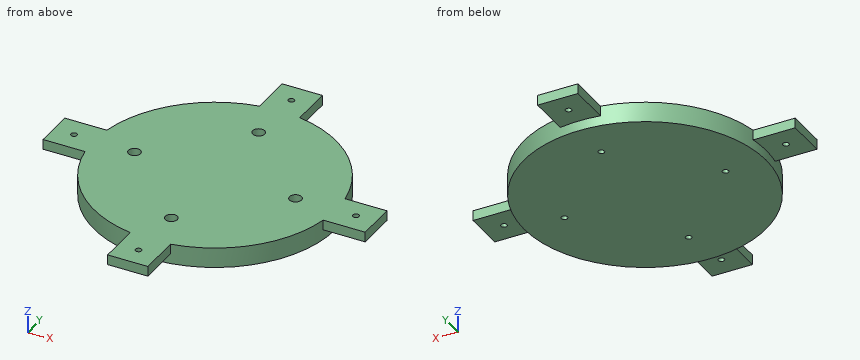
```python
from build123d import *

# Parameters (mm, degrees)
SKETCH1_R           = 60
BOSS_EXTRUDE1_DEPTH = 5
SKETCH3_W           = 20
SKETCH3_H           = 30
SKETCH3_W_2         = 30
SKETCH3_H_2         = 20
BOSS_EXTRUDE2_DEPTH = 5
SKETCH6_R           = 60
BOSS_EXTRUDE3_DEPTH = 10
SKETCH7_R           = 70
CUT_EXTRUDE2_DEPTH  = 5
SKETCH8_R           = 3
CUT_EXTRUDE7_DEPTH  = 5
SKETCH13_R          = 1.5
CUT_EXTRUDE10_DEPTH = 10


with BuildPart() as part:
    # Sketch1 → Boss-Extrude1 (new body)
    with BuildSketch(Plane.XY):
        Circle(SKETCH1_R)
    extrude(amount=BOSS_EXTRUDE1_DEPTH)

    # Sketch3 → Boss-Extrude2 (add)
    with BuildSketch(Plane(origin=(0, 0, 0), x_dir=(-1, 0, 0), z_dir=(0, 0, -1))):
        with Locations((0, -65)):
            Rectangle(SKETCH3_W, SKETCH3_H)
        with Locations((0, 65)):
            Rectangle(SKETCH3_W, SKETCH3_H)
        with Locations((65, 0)):
            Rectangle(SKETCH3_W_2, SKETCH3_H_2)
        with Locations((-65, 0)):
            Rectangle(SKETCH3_W_2, SKETCH3_H_2)
    extrude(amount=BOSS_EXTRUDE2_DEPTH)

    # Sketch6 → Boss-Extrude3 (add)
    with BuildSketch(Plane(origin=(0, 0, 0), x_dir=(-1, 0, 0), z_dir=(0, 0, -1))):
        Circle(SKETCH6_R)
    extrude(amount=BOSS_EXTRUDE3_DEPTH)

    # Sketch7 → Cut-Extrude2 (cut)
    with BuildSketch(Plane.XY.offset(5)):
        Circle(SKETCH7_R)
    extrude(amount=-CUT_EXTRUDE2_DEPTH, mode=Mode.SUBTRACT)

    # Sketch8 → Cut-Extrude7 (cut)
    with BuildSketch(Plane.XY):
        with Locations((0, -40)):
            Circle(SKETCH8_R)
        with Locations((0, 40)):
            Circle(SKETCH8_R)
        with Locations((-40, 0)):
            Circle(SKETCH8_R)
        with Locations((40, 0)):
            Circle(SKETCH8_R)
    extrude(amount=-CUT_EXTRUDE7_DEPTH, mode=Mode.SUBTRACT)

    # Sketch13 → Cut-Extrude10 (cut)
    with BuildSketch(Plane.XY):
        with Locations((-40, 0)):
            Circle(SKETCH13_R)
        with Locations((40, 0)):
            Circle(SKETCH13_R)
        with Locations((-70, 0)):
            Circle(SKETCH13_R)
        with Locations((70, 0)):
            Circle(SKETCH13_R)
        with Locations((0, -40)):
            Circle(SKETCH13_R)
        with Locations((0, -70)):
            Circle(SKETCH13_R)
        with Locations((0, 40)):
            Circle(SKETCH13_R)
        with Locations((0, 70)):
            Circle(SKETCH13_R)
    extrude(amount=-CUT_EXTRUDE10_DEPTH, mode=Mode.SUBTRACT)


solid = part.part
```
The model under review builds one solid part; all positions refer to its coordinate system, in mm. Round coordinates to 2 decimals unless told otherwise and drop trailing zeros. Order: outer loops, then holes, each group sorted by start corner. A loop starts at its lowest first (then second) coordinate and runs counter-clockwise, first axis right, second up. Notation, with made-up numbers: (-6.5, -30) -> (10.5, -30) arc R32 ccw to (10.5, 7) -> close; hole circle Ø7 at (61, 9). An arc over 180 degrees is marked (long way). Use a Markdown table: item, result.
Q1. We need section A-A on z = -7.5. Write out the cut boundary in (x, y), then the cut area to 3 significant figures.
Values:
| item | result |
|---|---|
| outline | circle Ø120 at (0, 0); hole circle Ø3 at (-40, 0); hole circle Ø3 at (0, -40); hole circle Ø3 at (0, 40); hole circle Ø3 at (40, 0) |
| area | 11,300 mm^2 |
Q2. For line 1 (X direction, y = 70, z = -3.1); line 2 (Y direction, x = 2.5, z = -2.25), list the stretches that pass through material, from the lowest coordinate up.
Values:
| item | result |
|---|---|
| line 1 | x = -10 to -1.5, 1.5 to 10 |
| line 2 | y = -80 to -41.66, -38.34 to 38.34, 41.66 to 80 |
Q3. Clearance check with flat-ended pins moving along their axes: P1, Ø4, axis at x = -32.5, z = -7, coming from the -Y side; P2, Ø16, axis at x = -70.5, y = 1, coming from the -Z side; P3, Ø5, axis at x = 26.5, z = -1, coming from the +Y side. State where each tip first meets the part, or that it passes through.
Values:
| item | result |
|---|---|
| P1 | stops at y = -51.67 |
| P2 | stops at z = -5 |
| P3 | stops at y = 54.99 |
Q4. We need section D-D on y = -24.5. Write out the cut boundary in (x, z).
Values:
| item | result |
|---|---|
| outline | (-54.77, -10) -> (54.77, -10) -> (54.77, 0) -> (-54.77, 0) -> close |
Q5. We need section B-B on y = -5.5. Write out the cut boundary in (x, z).
Values:
| item | result |
|---|---|
| outline | (-80, -5) -> (-59.75, -5) -> (-59.75, -10) -> (59.75, -10) -> (59.75, -5) -> (80, -5) -> (80, 0) -> (-80, 0) -> close |
Q6. We need section C-C on x = -8. Write out the cut boundary in (y, z).
Values:
| item | result |
|---|---|
| outline | (-80, -5) -> (-59.46, -5) -> (-59.46, -10) -> (59.46, -10) -> (59.46, -5) -> (80, -5) -> (80, 0) -> (-80, 0) -> close |
